Geometry check sheet. Reference: drawing and pictorial views, mm from the part's lowest x, y, z. A direction names the side the tool comes from. Round coordinates to 2 decimals unless told otherwise and drop trailing zeros. Write each loop counter-clockwise with the first axis right and the second up, starting at its lowest first coordinate (ties: lowest second). Pieces come first, ordered by that corner, then holes.
Item 1: Section check A-A, the plane x = 20. Record the cut outline in (y, z) (3 decimals).
Item 2: Section check C-C, the plane y = 22. Record the cut outline in (x, z) (3 decimals).
Item 3: Material ranges on line 1 along Y through (x, z) = (4.75, 3); line 2 along Y through (x, z) = (26.5, 4.2) (3 decimals); line 3 along X through (y, z) = (21.5, 2.25) (3 decimals), recorded low to high.
Item 4: Set-up check for the marked faces 4 and 5: record each of +Z, -Z, +X, -X, +Y, -Y from which the full face is reachable in a straight line by a thin tool's end or side.
Item 5: Section check D-D, the plane y = 36. Record the cut outline in (x, z), plus the area to 3 significant figures.
Item 6: Depth check by flat-ended pin: pin 1 (0.7 mm diameter, centred on y = 6.5, z = 2.5, fed in from +X); pin 2 (1.4 mm diameter, centred on y = 36, z = 3, fed in from -X); pin 3 (8 mm diameter, centred on x = 32.5, y = 22, fed in from +Z). Enter the tip coordinate at first touch or a pass-through.
Item 7: Section check B-B, the plane z = 3. Record the cut outline in (x, y) (3 decimals), plus the area to 3 significant figures.
Item 8: Release check for a two-part mould opening along Y. For the marked faces 1, 2 and 3 record: pulls with the +Y half, pulls with the -Y half, needs draft (parallel to the pull), parting line crosses it, or undercut.
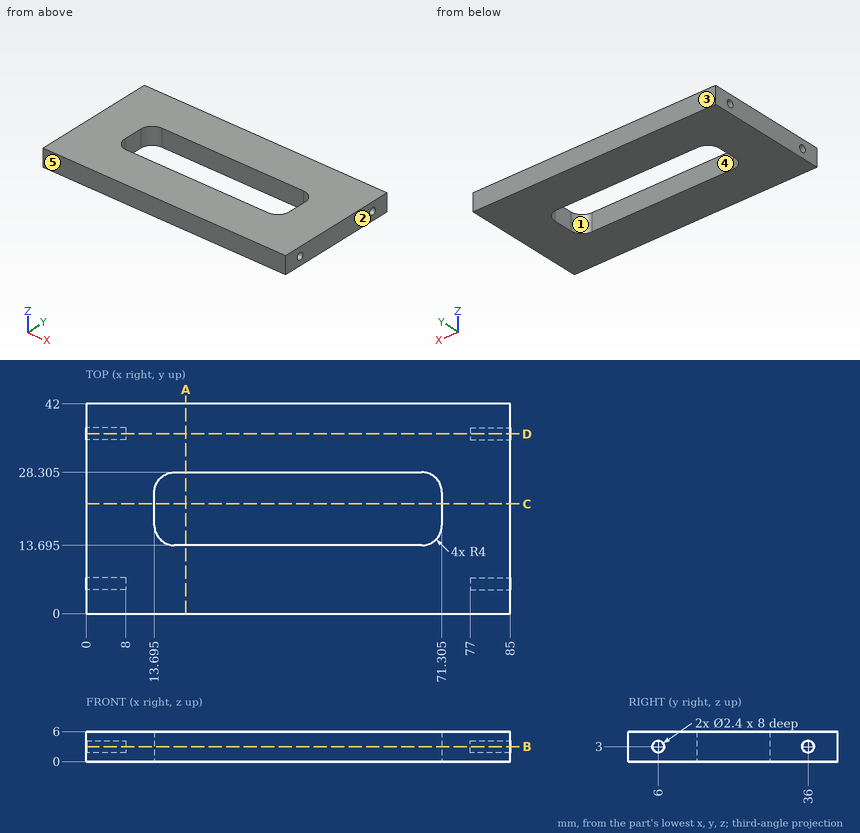
Values found:
1. outline: (0, 0) - (13.695, 0) - (13.695, 6) - (0, 6) - close; (28.305, 0) - (42, 0) - (42, 6) - (28.305, 6) - close
2. outline: (0, 0) - (13.695, 0) - (13.695, 6) - (0, 6) - close; (71.305, 0) - (85, 0) - (85, 6) - (71.305, 6) - close
3. line 1: y = 0 to 4.8, 7.2 to 34.8, 37.2 to 42
3. line 2: y = 0 to 13.695, 28.305 to 42
3. line 3: x = 0 to 13.695, 71.305 to 85
4. face 4: +Z, -Z
4. face 5: +Z, -Z, +X, -X, -Y
5. outline: (0, 0) - (85, 0) - (85, 1.8) - (77, 1.8) - (77, 4.2) - (85, 4.2) - (85, 6) - (0, 6) - (0, 4.2) - (8, 4.2) - (8, 1.8) - (0, 1.8) - close
5. area: 472 mm2
6. pin 1: stops at x = 77
6. pin 2: stops at x = 8
6. pin 3: passes through
7. outline: (0, 0) - (85, 0) - (85, 4.8) - (77, 4.8) - (77, 7.2) - (85, 7.2) - (85, 34.8) - (77, 34.8) - (77, 37.2) - (85, 37.2) - (85, 42) - (0, 42) - (0, 37.2) - (8, 37.2) - (8, 34.8) - (0, 34.8) - (0, 7.2) - (8, 7.2) - (8, 4.8) - (0, 4.8) - close; hole (13.695, 17.695) arc R4 ccw to (17.695, 13.695) - (67.305, 13.695) arc R4 ccw to (71.305, 17.695) - (71.305, 24.305) arc R4 ccw to (67.305, 28.305) - (17.695, 28.305) arc R4 ccw to (13.695, 24.305) - close
7. area: 2,670 mm2
8. face 1: undercut
8. face 2: needs draft
8. face 3: pulls with the +Y half
